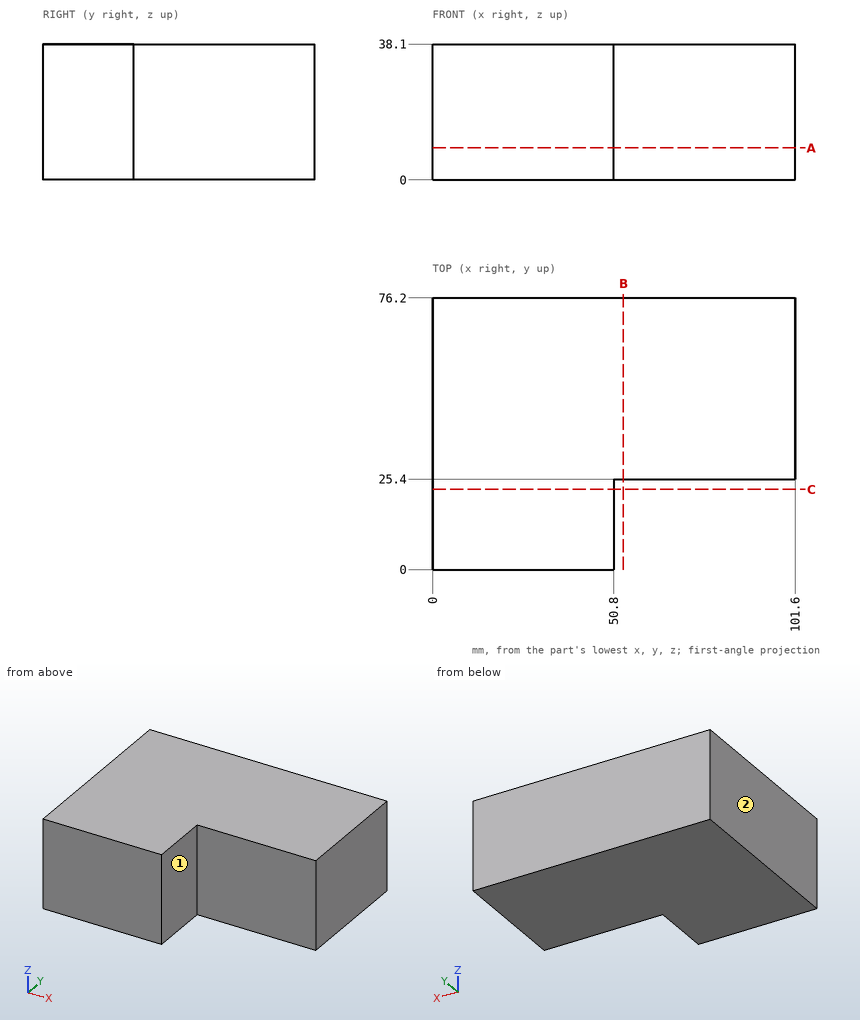
Can you work these out from the drawing? Everything is in mm from the part's minimum corner. A direction names the side the tool comes from. Give positions to 0.01 mm unless a question says otherwise; leave off trailing zeros. Order: outer loops, then holes, each group sorted by start corner. A loop starts at its lowest first (then second) coordinate and runs counter-clockwise, first axis right, second up. Notation, with made-up numbers: M -14.75,64 L -0.75,64 A10 cw -0.75,77 Z; hole C 1.5,83 d3. An arc over 180 degrees is marked long. Use a Markdown table: item, result. Add a question column.
1. Suppose I cut it at C-C (y = 22.5). List the corners of the cut face in (x, z) for me.
2. For pin 1 Ø12.5 at (y, z) = (9, 27) entering from +X; pin 2 Ø19 at (x, z) = (76.5, 21.5) entering from -Y, each with a flat end and sliding along its axis, tell me the tip position at first contact or that it passes through.
3. Suppose I cut it at A-A (z = 9). List the corners of the cut face in (x, y) for me.
4. Suppose I cut it at B-B (x = 53.5). List the corners of the cut face in (y, z) for me.
5. I need wall thicknesses on probe 1 along Y at (x, z) = (76, 20.5); probe 2 along X at (y, z) = (13, 5.5). Which ranges of each line are inside material? Lowest first, please. Write a range as from..to.
6. On a 3-axis mill with a long thin cutter (end or side, diameter ignored), from which of +Z, -Z, +X, -X, +Y, -Y can I reach the whole of each face in a straight line? I mean the marked faces 1 and 2. Say none if no direction works.
Results list:
| question | item | result |
|---|---|---|
| 1 | outline | M 0,0 L 50.8,0 L 50.8,38.1 L 0,38.1 Z |
| 2 | pin 1 | stops at x = 50.8 |
| 2 | pin 2 | stops at y = 25.4 |
| 3 | outline | M 0,0 L 50.8,0 L 50.8,25.4 L 101.6,25.4 L 101.6,76.2 L 0,76.2 Z |
| 4 | outline | M 25.4,0 L 76.2,0 L 76.2,38.1 L 25.4,38.1 Z |
| 5 | probe 1 | y = 25.4..76.2 |
| 5 | probe 2 | x = 0..50.8 |
| 6 | face 1 | +Z, -Z, +X, -Y |
| 6 | face 2 | +Z, -Z, -X, +Y, -Y |
